CAD build for the part. Positions are in the model's coordinates, mm. Coordinates: 2 decimals unless noted, no trailing zeros. Write each loop counter-clockwise with the first axis right and the second up, starting at its lowest first coordinate (ties: lowest second). Pieces come first, ordered by that corner, then holes. Notation, with made-up numbers: M 19.5,89 L 27.5,89 A21 cw 27.5,111 Z; hole C 19,14.5 d4. An arc over 180 degrees is marked long. Put each result on its own line as item: value. Start each with the question number.
```python
from build123d import *

# Parameters (mm, degrees)
BOSS_EXTRUDE1_DEPTH              = 20
F_10_0MM_DOWEL_HOLE1_D           = 10
F_10_0MM_DOWEL_HOLE1_DEPTH       = 20
F_10_0MM_DOWEL_HOLE1_CSINK_D     = 10.05
F_10_0MM_DOWEL_HOLE1_CSINK_ANGLE = 90


with BuildPart() as part:
    # Sketch1 → Boss-Extrude1 (new body)
    with BuildSketch(Plane.XY):
        with BuildLine():
            Line((0, 0), (0, 480))
            ThreePointArc((0, 480), (10, 490), (20, 480))
            Line((20, 480), (20, 0))
            ThreePointArc((20, 0), (10, -10), (0, 0))
        make_face()
    extrude(amount=BOSS_EXTRUDE1_DEPTH)

    # Ø10.0mm Dowel Hole1
    with Locations(Plane.XY.offset(20)):
        with Locations((10, 480), (10, 0)):
            CounterSinkHole(F_10_0MM_DOWEL_HOLE1_D / 2, F_10_0MM_DOWEL_HOLE1_CSINK_D / 2, depth=F_10_0MM_DOWEL_HOLE1_DEPTH, counter_sink_angle=F_10_0MM_DOWEL_HOLE1_CSINK_ANGLE)


solid = part.part
```
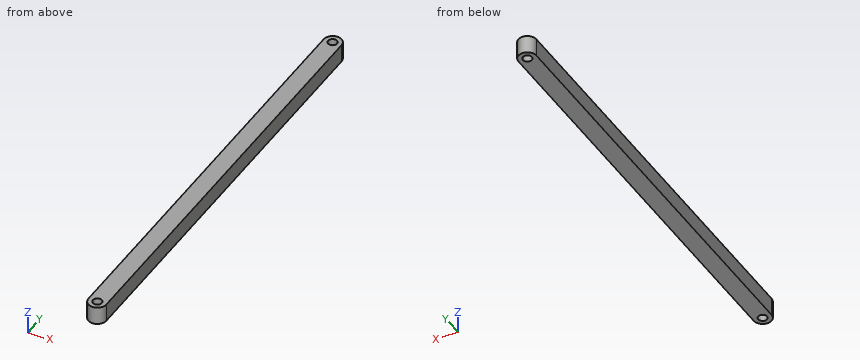
(1) Slice it at A-A, the plane x = 10. Write the cut outline in (y, z) (3 decimals), then the cut area to 3 significant figures.
(2) Drill centre lines: line 1 (X direction, y = 480, z = 11.75); line 2 (Y direction, x = 7, z = 4.25); line 3 (Y direction, x = 6.75, z = 1). Where is each one in solid material? Low to high. Write a range as [from, to].
(3) Slice it at B-B, the plane z = 7. Write the cut outline in (x, y), then the cut area to 3 significant figures.
(4) Drop flat-ended pins along their axis: pin 1 (5 mm diameter, centred on x = 2.5, z = 13.5, fed in from -Y); pin 2 (10 mm diameter, centred on x = 18, z = 15.5, fed in from -Y). Give the stop position or say it passes through.
Result set:
1. outline: M -10,0 L -5,0 L -5,19.975 L -5.025,20 L -10,20 Z; M 5,0 L 475,0 L 475,19.975 L 474.975,20 L 5.025,20 L 5,19.975 Z; M 485,0 L 490,0 L 490,20 L 485.025,20 L 485,19.975 Z
1. area: 9,600 mm^2
2. line 1: x = [0, 5], [15, 20]
2. line 2: y = [-9.54, -4], [4, 476], [484, 489.54]
2. line 3: y = [-9.46, -3.8], [3.8, 476.2], [483.8, 489.46]
3. outline: M 0,0 A10 ccw 20,0 L 20,480 A10 ccw 0,480 Z; hole C 10,0 d10; hole C 10,480 d10
3. area: 9,760 mm^2
4. pin 1: stops at y = -8.66
4. pin 2: stops at y = -9.54
